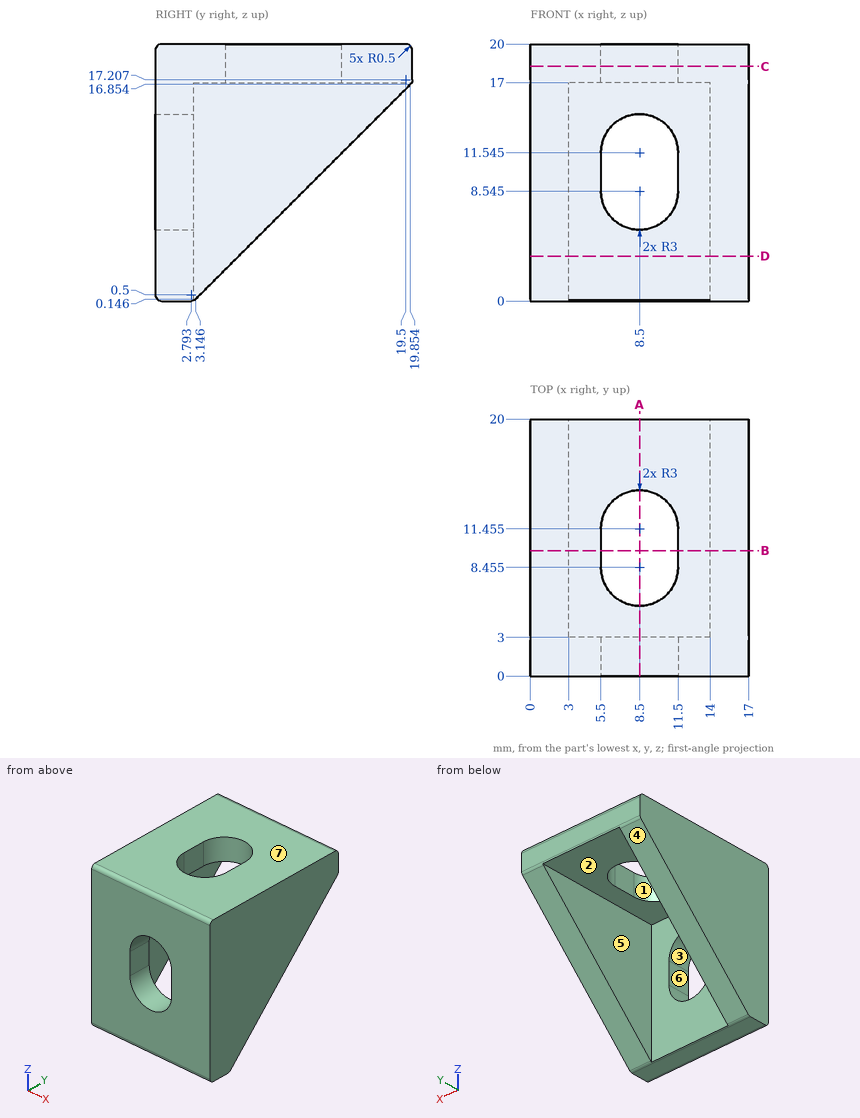
Job drawing, mm, ordinate dimensions from the low corner. One solid piece. A direction names the side the tool comes from. Round coordinates to 2 decimals unless told otherwise and drop trailing zeros. Loops run counter-clockwise (first coordinate to the right, second up) from the corner with the lowest first, then second, coordinate; pieces in that order, holes last.
(1) Wall check: line 1 along X through (y, z) = (7.75, 5.25); line 2 along Y through (x, z) = (4.5, 14.5); line 3 along Z through (x, y) = (7.25, 16.5). Give the ranges that are in metal, low to high.
(2) Cut at A-A (x = 8.5). State how many separate pieces and enclosed holes the cut face has.
(3) Two-plate mould, pull along Z, no slides. Class the marked faces 4, 5, 6 and 7: +Z half, -Z half, draft (parallel to the pull), parting line (faces both ways), or undercut.
(4) Drop flat-ended pins along their axis: pin 1 (2 mm diameter, centred on x = 6, z = 7, fed in from +Y); pin 2 (5.5 mm diameter, centred on x = 10.5, y = 14, fed in from -Z); pin 3 (6 mm diameter, centred on x = 13.5, y = 15.5, fed in from -Z). Give the stop position or say it passes through.
(5) Cut at B-B (y = 9.75). Give the cut face in (x, z).
(6) Which spindle directions (+Z, -Z, +X, -X, +Y, -Y) get a long thin tool onto all of the face, cutting with end or side? Do the marked faces 1, 2 and 3. Say none if no direction does.
(7) Cut at C-C (z = 18.25). Give the cut face in (x, y) (1 decimal), plus the area to 3 significant figures.
(8) Cut at D-D (z = 3.5). Give the cut face in (x, y), plus the area to 3 significant figures.
Findings below:
1. line 1: x = 0 to 3, 14 to 17
1. line 2: y = 0 to 3
1. line 3: z = 17 to 20
2. separate pieces: 3
2. enclosed holes: 0
3. face 4: -Z half
3. face 5: draft
3. face 6: undercut
3. face 7: +Z half
4. pin 1: stops at y = 3
4. pin 2: stops at z = 17
4. pin 3: stops at z = 9.54
5. outline: (0, 6.75) - (3, 6.75) - (3, 17) - (5.5, 17) - (5.5, 20) - (0, 20) - close; (11.5, 17) - (14, 17) - (14, 6.75) - (17, 6.75) - (17, 20) - (11.5, 20) - close
6. face 1: +Z, -Z
6. face 2: -Z, +Y
6. face 3: +Y, -Y
7. outline: (0, 0) - (17, 0) - (17, 20) - (0, 20) - close; hole (5.5, 8.5) arc R3 ccw to (11.5, 8.5) - (11.5, 11.5) arc R3 ccw to (5.5, 11.5) - close
7. area: 294 mm2
8. outline: (0, 0) - (17, 0) - (17, 6.5) - (14, 6.5) - (14, 3) - (3, 3) - (3, 6.5) - (0, 6.5) - close
8. area: 72.0 mm2
